Verification items for the finished model (mm, model axes). Face numbers are marked on the shaded views. Give positions to 0.01 mm unless a question says otherwise; leave off trailing zeros. Order: outer loops, then holes, each group sorted by start corner. A loop starts at its lowest first (then second) coordinate and runs counter-clockwise, first axis right, second up.
(1) Sectioned sample at B-B on z = 0. Record the cut outline in (x, y).
(2) Gauge pin test, flat end, axial feed: pin 1 (1.5 mm diameter, centred on x = -1.5, y = 2.5, fed in from -Z). Record the tip position at first contact, or that the pin passes through.
(3) Scan lines: L1, parallel to Z at x = 0, y = -1.85 (3 decimals); L2, parallel to X at y = 1.55, z = 0; L3, parallel to Z at x = -3.25, y = 3. Record each from-to range of solid material in increasing order.
(4) Mould release check, pull along Y, two halves, no side actions. Record for the marked faces 1, 2 and 3: pulls with the +Y half, pulls with the -Y half, needs draft (parallel to the pull), parting line crosses it, or undercut.
```python
from build123d import *

# Parameters (mm, degrees)
SKETCH2_R                = 4
BOSS_EXTRUDE1_DEPTH      = 3.25
BOSS_EXTRUDE1_DEPTH_BACK = 3.25
FILLET1_R                = 0.65
CUT_EXTRUDE2_DEPTH       = 0.25


with BuildPart() as part:
    # Sketch2 → Boss-Extrude1 (new body, two sides)
    with BuildSketch(Plane(origin=(0, 0, 0), x_dir=(1, 0, 0), z_dir=(0, 1, 0))) as boss_extrude1_sk:
        Polygon((0, 7.505553499), (-6.5, 3.75277675), (-6.5, -3.75277675), (0, -7.505553499), (6.5, -3.75277675), (6.5, 3.75277675), align=None)
        Circle(SKETCH2_R, mode=Mode.SUBTRACT)
    extrude(amount=BOSS_EXTRUDE1_DEPTH)
    extrude(boss_extrude1_sk.sketch, amount=-BOSS_EXTRUDE1_DEPTH_BACK)

    # Fillet1
    fillet1_edges = [part.edges().sort_by_distance(p)[0] for p in [
        (6.5, 0, -3.75277675),
        (6.5, 0, 3.75277675),
        (0, 0, 7.505553499),
        (-6.5, 0, 3.75277675),
        (-6.5, 0, -3.75277675),
        (0, 0, -7.505553499),
    ]]
    fillet(fillet1_edges, radius=FILLET1_R)

    # Sketch3 → Cut-Revolve2 (revolve, cut)
    with BuildSketch(Plane(origin=(0, 0, 0), x_dir=(0, 0, -1), z_dir=(1, 0, 0))):
        Polygon((6.3375, -3.25), (7.505553499, -2.575623998), (7.505553499, -3.25), align=None)
        Polygon((4, 3.25), (4, 3.05), (4.2, 3.25), align=None)
        Polygon((4, -3.25), (4, -3.05), (4.2, -3.25), align=None)
        Polygon((6.3375, 3.25), (7.505553499, 2.575623998), (7.505553499, 3.25), align=None)
    revolve(axis=Axis((0, -3.25, 0), (0, 1, 0)), mode=Mode.SUBTRACT)

    # Sketch12 → Cut-Extrude2 (cut)
    with BuildSketch(Plane(origin=(3.25, 0, 5.629165125), x_dir=(0.866025404, 0, -0.5), z_dir=(0.5, 0, 0.866025404))):
        Polygon((-1.214814445, 0), (-0.607407223, -1.05206017), (0.607407223, -1.05206017), (1.214814445, 0), (0.607407223, 1.05206017), (-0.607407223, 1.05206017), align=None)
    extrude(amount=-CUT_EXTRUDE2_DEPTH, mode=Mode.SUBTRACT)


solid = part.part
```
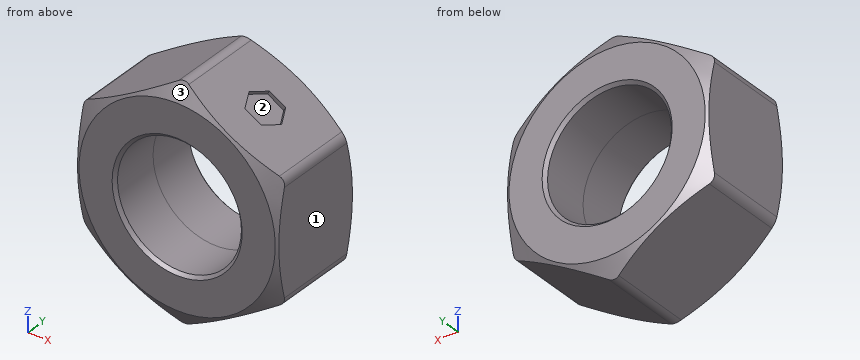
Ans:
1. outline: (-6.5, -3.16) - (-6.34, -3.25) - (-4.2, -3.25) - (-4, -3.05) - (-4, 3.05) - (-4.2, 3.25) - (-6.34, 3.25) - (-6.5, 3.16) - close; (4, -3.05) - (4.2, -3.25) - (6.34, -3.25) - (6.5, -3.16) - (6.5, 3.16) - (6.34, 3.25) - (4.2, 3.25) - (4, 3.05) - close
2. pin 1: stops at z = -7.07
3. L1: z = -7.405 to -4, 4 to 7.405
3. L2: x = -6.5 to -4, 4 to 6.5
3. L3: z = -5.63 to -2.33, 2.33 to 5.63
4. face 1: needs draft
4. face 2: undercut
4. face 3: pulls with the -Y half
